The drawing under review shows one solid part. Ordinate dimensions are in mm from its lowest x, y, z. Round coordinates to 2 decimals unless told otherwise and drop trailing zeros. Order: outer loops, then holes, each group sorted by start corner. A loop starts at its lowest first (then second) coordinate and runs counter-clockwise, first axis right, second up. Notation, with made-up numbers: M 50,56 L 97,56 A15 ccw 97,70 Z; hole C -36,68.25 d11. An arc over 180 degrees is marked long. Write item = value, one per line. Start each with the question number.
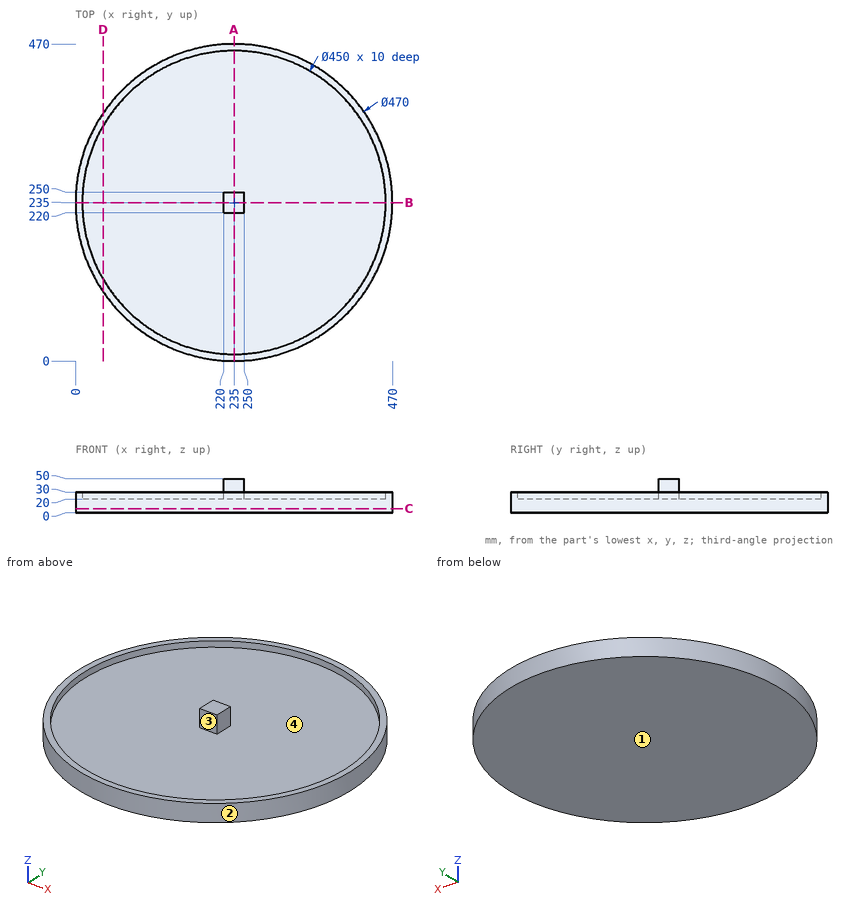
(1) Consider section C-C, the plane z = 6. Write out the cut boundary in (x, y).
(2) Draft analysis for pull direction X (two halves, no side actions). For the marked faces 1, 2, 3 and 4, state which applies: pulls with the +X half, pulls with the -X half, needs draft (parallel to the pull), parting line crosses it, or undercut.
(3) Consider section D-D, the plane x = 41. Write out the cut boundary in (y, z), then the cut area to 3 significant figures.
(4) Insertion check: pin 1 (12 mm diameter, centred on x = 195, z = 18, fed in from +Y); pin 2 (8 mm diameter, centred on x = 266.5, z = 18.5, fed in from +Y); pin 3 (6 mm diameter, centred on y = 376.5, z = 30.5, fed in from -X). Each pin has a flat end and moves straight along its axis. Give the tip position at first contact, or say it passes through.
(5) Consider section A-A, the plane x = 235. Write out the cut boundary in (y, z).
(6) For line 1 along Y through (x, z) = (235, 27); line 2 along Z through (x, y) = (170, 247); line 3 along X through (y, z) = (199.5, 21.5), list the stretches that pass through material, from the lowest coordinate up. Write a range as [from, to].
Completed:
q1.outline = C 235,235 d470
q2.face_1 = needs draft
q2.face_2 = parting line crosses it
q2.face_3 = undercut
q2.face_4 = undercut
q3.outline = M 102.38,0 L 367.62,0 L 367.62,30 L 348.97,30 L 348.97,20 L 121.03,20 L 121.03,30 L 102.38,30 Z
q3.area = 5,680 mm2
q4.pin_1 = 467.53
q4.pin_2 = 468.39
q4.pin_3 = 45.18
q5.outline = M 0,0 L 470,0 L 470,30 L 460,30 L 460,20 L 250,20 L 250,50 L 220,50 L 220,20 L 10,20 L 10,30 L 0,30 Z
q6.line_1 = [0, 10], [220, 250], [460, 470]
q6.line_2 = [0, 20]
q6.line_3 = [2.7, 12.82], [457.18, 467.3]
